Model file for the job. Use its own axes, mm. Face numbers are marked on the shaded views. A direction names the side the tool comes from. Round coordinates to 2 decimals unless told otherwise and drop trailing zeros. Order: outer loops, then holes, each group sorted by start corner. A loop starts at its lowest first (then second) coordinate and runs counter-clockwise, first axis right, second up. Notation, with made-up numbers: (-36, 50.25) -> (-21, 50.25) arc R19 ccw to (-21, 78.25) -> close; hole circle Ø5 at (88.25, 3.5). An arc over 180 degrees is marked (long way). Answer as CSV lines item,"result".
```python
from build123d import *

# Parameters (mm, degrees)
F1_DEPTH = 10
F2_R     = 2.5
F3_DEPTH = 25
F5_DEPTH = 3
F7_DEPTH = 3


with BuildPart() as f1:
    # F0 (on Front) → F1 (new body, symmetric)
    with BuildSketch(Plane.XZ):
        with BuildLine():
            ThreePointArc((-12.3133069376, 2.1523178808), (0, 12.5), (12.3133069376, 2.1523178808))
            ThreePointArc((12.3133069376, 2.1523178808), (13.2017484895, 0.6095259974), (14.8744747806, 0))
            Line((14.8744747806, 0), (29.85, 0))
            Line((29.85, 0), (29.85, 3))
            Line((29.85, 3), (16.503, 3))
            ThreePointArc((16.503, 3), (15.7100109406, 3.2698697404), (15.2462584222, 3.9674333051))
            ThreePointArc((15.2462584222, 3.9674333051), (9.6127418909, 12.3640200256), (0, 15.5))
            ThreePointArc((0, 15.5), (-9.6127418909, 12.3640200256), (-15.2462584222, 3.9674333051))
            ThreePointArc((-15.2462584222, 3.9674333051), (-15.7100109406, 3.2698697404), (-16.503, 3))
            Line((-16.503, 3), (-29.85, 3))
            Line((-29.85, 3), (-29.85, 0))
            Line((-29.85, 0), (-14.8744747806, 0))
            ThreePointArc((-14.8744747806, 0), (-13.2017484895, 0.6095259974), (-12.3133069376, 2.1523178808))
        make_face()
    extrude(amount=F1_DEPTH, both=True)

    # F2 (on face) → F3 (cut)
    with BuildSketch(Plane.XY.offset(3)):
        with Locations((-24.92, 0)):
            Circle(F2_R)
        with Locations((24.92, 0)):
            Circle(F2_R)
    extrude(amount=-F3_DEPTH, mode=Mode.SUBTRACT)

    # F4 (on face) → F5 (join)
    with BuildSketch(Plane.XY.offset(3)):
        with BuildLine():
            Line((-29.85, -10), (-29.85, 10))
            ThreePointArc((-29.85, 10), (-33.7754930507, 0), (-29.85, -10))
        make_face()
    extrude(amount=-F5_DEPTH)

    # F6 (on face) → F7 (join)
    with BuildSketch(Plane.XY.offset(3)):
        with BuildLine():
            Line((29.85, 10), (29.85, -10))
            ThreePointArc((29.85, -10), (33.7754930507, 0), (29.85, 10))
        make_face()
    extrude(amount=-F7_DEPTH)


solid = f1.part
```
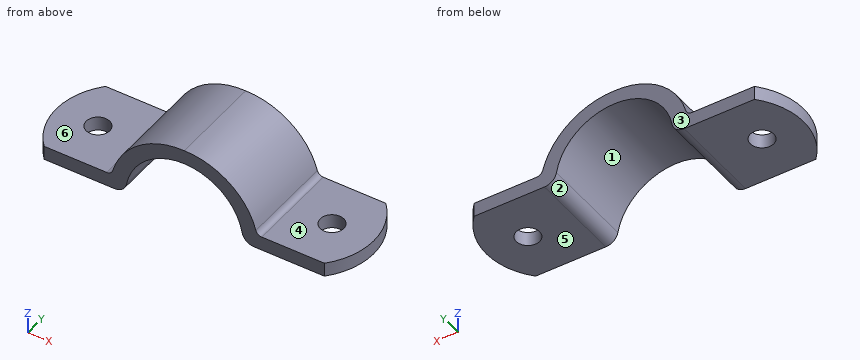
Q1. Saw through at D-D (y = -4.5). Write the cut outline in (x, z).
Checks:
outline,"(-33.07, 0) -> (-14.87, 0) arc R2.6 ccw to (-12.31, 2.15) arc R12.5 cw to (12.31, 2.15) arc R2.6 ccw to (14.87, 0) -> (33.07, 0) -> (33.07, 3) -> (16.5, 3) arc R1.3 cw to (15.25, 3.97) arc R15.5 ccw to (0, 15.5) arc R15.5 ccw to (-15.25, 3.97) arc R1.3 cw to (-16.5, 3) -> (-33.07, 3) -> close"
Q2. Saw through at C-C (z = 11.75). Write the cut outline in (x, y).
Checks:
outline,"(-10.37, -10) -> (-4.26, -10) -> (-4.26, 10) -> (-10.37, 10) -> close; (4.26, -10) -> (10.37, -10) -> (10.37, 10) -> (4.26, 10) -> close"
Q3. Saw through at B-B (y = 0). Write the cut outline in (x, z).
Checks:
outline,"(-33.78, 0) -> (-27.42, 0) -> (-27.42, 3) -> (-33.78, 3) -> close; (-22.42, 0) -> (-14.87, 0) arc R2.6 ccw to (-12.31, 2.15) arc R12.5 cw to (12.31, 2.15) arc R2.6 ccw to (14.87, 0) -> (22.42, 0) -> (22.42, 3) -> (16.5, 3) arc R1.3 cw to (15.25, 3.97) arc R15.5 ccw to (0, 15.5) arc R15.5 ccw to (-15.25, 3.97) arc R1.3 cw to (-16.5, 3) -> (-22.42, 3) -> close; (27.42, 0) -> (33.78, 0) -> (33.78, 3) -> (27.42, 3) -> close"
Q4. Mould opens along X. For the marked faces 1, 2 and 3 say: +X half, -X half, draft (parallel to the pull), parting line (faces both ways), or undercut.
Checks:
face 1,"undercut"
face 2,"undercut"
face 3,"draft"
Q5. Saw through at A-A (x = -24.92). Write the cut outline in (y, z), plus the area to 3 significant figures.
Checks:
outline,"(-10, 0) -> (-2.5, 0) -> (-2.5, 3) -> (-10, 3) -> close; (2.5, 0) -> (10, 0) -> (10, 3) -> (2.5, 3) -> close"
area,"45.0 mm²"
Q6. Tool access for the marked faces 4, 5 and 6: list every direction of +Z, -Z, +X, -X, +Y, -Y with a clear straight run to the whole face (end or side of a thin tool).
Checks:
face 4,"+Z, +X, +Y, -Y"
face 5,"-Z, +X, -X, +Y, -Y"
face 6,"+Z, -X, +Y, -Y"
Q7. Wall check: L1, parallel to X at y = 0.75, z = 1; L2, parallel to Y at x = 24.92, z = 1.85; L3, parallel to Z at x = 18.5, y = -5.5. Give the ranges that are in metal, low to high. Write a range as [from, to].
Checks:
L1,"[-33.76, -27.3], [-22.54, -12.83], [12.83, 22.54], [27.3, 33.76]"
L2,"[-10, -2.5], [2.5, 10]"
L3,"[0, 3]"
Q8. Flat gauge pins, fed straight in: pin 1 (3 mm diameter, centred on x = -24.92, y = 0, fed in from -Z); pin 2 (8.5 mm diameter, centred on x = 29, y = 2, fed in from +Z); pin 3 (2 mm diameter, centred on y = -3, z = 9, fed in from -X). Where does each tip first touch, or does it go through?
Checks:
pin 1,"through"
pin 2,"z = 3"
pin 3,"x = -13.54"
